Part model, mm, in its own coordinate system. A direction names the side the tool comes from. Coordinates: 2 decimals unless noted, no trailing zeros. Loops run counter-clockwise (first coordinate to the right, second up) from the corner with the lowest first, then second, coordinate; pieces in that order, holes last. Notation, with made-up numbers: M -25,54 L 12,54 A19 cw 12,68 Z; hole C -19,67.5 d3. An arc over 180 degrees is marked long. Answer as a JSON object with one key per item and string values. Group by question number.
1. Saw through at A-A on y = 21. Write the cut outline in (x, z).
2. Saw through at D-D on y = 4. Write the cut outline in (x, z), then the cut area to 3 significant figures.
3. 3-axis set-ups, long thin cutter, end or side, ignore diameter. For faces 5 (the face through (12.7, 19, 32)), 6 (the face through (19, 6, 25.254)), 7 (the face through (10, 0, 23)), 8 (the face through (6, 12.7, 19)): which of +Z, -Z, +X, -X, +Y, -Y reach the whole face in a straight line?
4. Drill centre lines: L1, parallel to Y at x = 21.5, z = 25.5; L2, parallel to Z at x = 22, y = 10.5. Where is each one in solid material? Low to high.
5. Drop flat-ended pins along their axis: pin 1 Ø7.5 at (y, z) = (17.5, 15) entering from +X; pin 2 Ø4 at (x, z) = (13.5, 23) entering from +Y; pin 3 Ø6.5 at (x, y) = (18, 7.5) entering from -Z; pin 4 Ø10 at (x, y) = (5.5, 20.5) entering from -Z. Give the stop position or say it passes through.
6. Saw through at B-B on x = 3. Write the cut outline in (y, z).
7. Mould opens along Z. For faces 1 (the face through (6, 13, 0)), 2 (the face through (10, 10, 37.954)), 3 (the face through (6, 19, 12.554)), 4 (the face through (25.4, 6, 32)) say: released by +Z, released by -Z, zero draft, split by the parting line, or undercut.
8. Saw through at C-C on z = 32.5. Write the cut outline in (x, y).
from build123d import *

# Parameters (mm, degrees)
F0_W     = 12.7
F0_H     = 12.7
F1_DEPTH = 25.4
F2_DEPTH = 12.7


with BuildPart() as f1:
    # F0 (on Right) → F1 (new body)
    with BuildSketch(Plane.YZ):
        with Locations((6.35, 31.6040249003)):
            Rectangle(F0_W, F0_H)
    extrude(amount=F1_DEPTH)

    # F0 (on Right) → F2 (join)
    with BuildSketch(Plane.YZ):
        Polygon((0, 25.2540249003), (0, 0), (25.4, 0), (25.4, 12.5540249003), (12.7, 12.5540249003), (12.7, 25.2540249003), align=None)
        with Locations((19.05, 31.6040249003)):
            Rectangle(F0_W, F0_H)
    extrude(amount=F2_DEPTH)


solid = f1.part
Outcome:
{
 "1": {"outline": "M 0,0 L 12.7,0 L 12.7,12.55 L 0,12.55 Z; M 0,25.25 L 12.7,25.25 L 12.7,37.95 L 0,37.95 Z"},
 "2": {"outline": "M 0,0 L 12.7,0 L 12.7,25.25 L 25.4,25.25 L 25.4,37.95 L 0,37.95 Z", "area": "643 mm²"},
 "3": {"face 5": "+Z, -Z, +X, +Y", "face 6": "-Z, +X, +Y, -Y", "face 7": "+Z, -Z, +X, -X, -Y", "face 8": "+X, -X, +Y"},
 "4": {"L1": "y = 0 to 12.7", "L2": "z = 25.25 to 37.95"},
 "5": {"pin 1": "stops at x = 12.7", "pin 2": "stops at y = 12.7", "pin 3": "stops at z = 25.25", "pin 4": "stops at z = 0"},
 "6": {"outline": "M 0,0 L 25.4,0 L 25.4,12.55 L 12.7,12.55 L 12.7,25.25 L 25.4,25.25 L 25.4,37.95 L 0,37.95 Z"},
 "7": {"face 1": "released by -Z", "face 2": "released by +Z", "face 3": "undercut", "face 4": "zero draft"},
 "8": {"outline": "M 0,0 L 25.4,0 L 25.4,12.7 L 12.7,12.7 L 12.7,25.4 L 0,25.4 Z"}
}
